The listing builds one solid part. Answer for the finished solid, in the listing's coordinates (mm). Face numbers are marked on the shaded views. A direction names the side the tool comes from. Round coordinates to 2 decimals unless told otherwise and drop trailing zeros. Order: outer loops, then holes, each group sorted by start corner. A loop starts at its lowest first (then second) coordinate and runs counter-clockwise, first axis right, second up. Notation, with made-up numbers: M 0.25,66.25 L 42.25,66.25 A28 ccw 42.25,92.25 Z; hole C 54.25,70.5 d7. An arc over 180 degrees is marked long. Put each result on its own line as item: value. Start each with the question number.
1. The part is cut by section D-D (z = 13). Give the vertices of the cut face in (x, y), then the cut area to 3 significant figures.
2. Which of the six approach directions +Z, -Z, +X, -X, +Y, -Y give full straight-line access (tool end or side, diameter ignored) to the marked faces 1, 2 and 3?
3. The part is cut by section B-B (x = 4). Give the vertices of the cut face in (y, z).
4. The mould has two halves that part along Y. Classify the marked faces 4, 5 and 6: +Y half, -Y half, draft (parallel to the pull), parting line (faces both ways), or undercut.
5. The part is cut by section A-A (z = 7). Give the vertices of the cut face in (x, y), then the cut area to 3 significant figures.
6. Consider line 1 (X direction, y = -12, z = 7); line 2 (Y direction, x = 2.25, z = 7); line 3 (X direction, y = 14.5, z = 12.75). Determine where each line is inside the solid, lowest interval first.
7. The part is cut by section C-C (y = 13). Give the vertices of the cut face in (x, z), then the cut area to 3 significant figures.
8. Each of these flat-tipped pins is pushed along its axis until it touches: pin 1 Ø4 at (x, z) = (23.01, 7) entering from -Y; pin 2 Ø6.5 at (y, z) = (14.35, 7) entering from +X; pin 3 Ø3 at (x, z) = (-5.5, 5) entering from +Y. Where does it stop, or does it pass through?
from build123d import *

# Parameters (mm, degrees)
SALIENTE_EXTRUIR1_DEPTH = 14
CROQUIS2_R              = 4.035649311
CORTAR_EXTRUIR1_DEPTH   = 14
CROQUIS5_R              = 2.497749653
CORTAR_EXTRUIR2_DEPTH   = 14
CROQUIS7_R              = 2.514867633
CORTAR_EXTRUIR3_DEPTH   = 14
CROQUIS8_W              = 1.02892534
CROQUIS8_H              = 10.439450899
CORTAR_EXTRUIR4_DEPTH   = 14
CROQUIS9_R              = 2.593975345
CORTAR_EXTRUIR5_DEPTH   = 30


with BuildPart() as part:
    # Croquis1 → Saliente-Extruir1 (new body)
    with BuildSketch(Plane.XY):
        Polygon((-2.000386176, 17.69916911), (15.999613824, 17.69916911), (15.999613824, -9.30083089), (26.999613824, -9.30083089), (26.999613824, -15.30083089), (15.999613824, -15.30083089), (-2.000386176, -15.30083089), (-13.000386176, -15.30083089), (-13.000386176, -9.30083089), (-2.000386176, -9.30083089), align=None)
    extrude(amount=SALIENTE_EXTRUIR1_DEPTH)

    # Croquis2 → Cortar-Extruir1 (cut)
    with BuildSketch(Plane.XY.offset(14)):
        with Locations((6.999613824, 4.803097651)):
            Circle(CROQUIS2_R)
    extrude(amount=-CORTAR_EXTRUIR1_DEPTH, mode=Mode.SUBTRACT)

    # Croquis5 → Cortar-Extruir2 (cut)
    with BuildSketch(Plane(origin=(0, -9.30083089, 0), x_dir=(1, 0, 0), z_dir=(0, 1, 0))):
        with Locations((-9.06576441, -7)):
            Circle(CROQUIS5_R)
    extrude(amount=-CORTAR_EXTRUIR2_DEPTH, mode=Mode.SUBTRACT)

    # Croquis7 → Cortar-Extruir3 (cut)
    with BuildSketch(Plane(origin=(0, -9.30083089, 0), x_dir=(1, 0, 0), z_dir=(0, 1, 0))):
        with Locations((23.014515722, -7)):
            Circle(CROQUIS7_R)
    extrude(amount=-CORTAR_EXTRUIR3_DEPTH, mode=Mode.SUBTRACT)

    # Croquis8 → Cortar-Extruir4 (cut)
    with BuildSketch(Plane.XY.offset(14)):
        with Locations((6.999613824, 13.435682)):
            Rectangle(CROQUIS8_W, CROQUIS8_H)
    extrude(amount=-CORTAR_EXTRUIR4_DEPTH, mode=Mode.SUBTRACT)

    # Croquis9 → Cortar-Extruir5 (cut, through all)
    with BuildSketch(Plane.ZY.offset(2.000386176)):
        with Locations((7, 14.351263228)):
            Circle(CROQUIS9_R)
    extrude(amount=-CORTAR_EXTRUIR5_DEPTH, mode=Mode.SUBTRACT)


solid = part.part
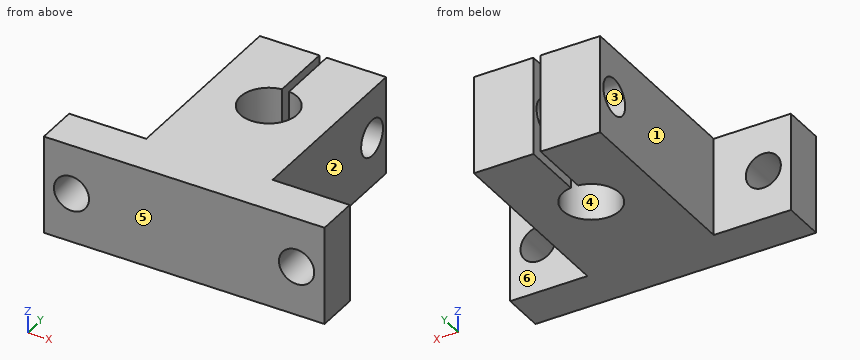
Resolved:
1. outline: M -13,-15.3 L 27,-15.3 L 27,-9.3 L 16,-9.3 L 16,17.7 L 7.51,17.7 L 7.51,8.81 A4.04 cw long 6.49,8.81 L 6.49,17.7 L -2,17.7 L -2,-9.3 L -13,-9.3 Z
1. area: 666 mm2
2. face 1: +Z, -Z, -X, +Y
2. face 2: +Z, -Z, +X, +Y
2. face 3: +X, -X
3. outline: M -15.3,0 L 2.1,0 L 2.1,14 L -15.3,14 Z; M 7.5,0 L 17.7,0 L 17.7,14 L 7.5,14 Z; hole C 14.35,7 d5.19
4. face 4: undercut
4. face 5: -Y half
4. face 6: +Y half
5. outline: M -13,-15.3 L -11.56,-15.3 L -11.56,-9.3 L -13,-9.3 Z; M -6.57,-15.3 L 20.5,-15.3 L 20.5,-9.3 L 16,-9.3 L 16,11.76 L 7.51,11.76 L 7.51,8.81 A4.04 cw long 6.49,8.81 L 6.49,11.76 L -2,11.76 L -2,-9.3 L -6.57,-9.3 Z; M -2,16.95 L 6.49,16.95 L 6.49,17.7 L -2,17.7 Z; M 7.51,16.95 L 16,16.95 L 16,17.7 L 7.51,17.7 Z; M 25.53,-15.3 L 27,-15.3 L 27,-9.3 L 25.53,-9.3 Z
5. area: 518 mm2
6. line 1: -13 to -11.56, -6.57 to 20.5, 25.53 to 27
6. line 2: -15.3 to 11.76, 16.95 to 17.7
6. line 3: -2 to 6.49, 7.51 to 16
7. outline: M -2,0 L 6.49,0 L 6.49,4.79 L -2,4.79 Z; M -2,9.21 L 6.49,9.21 L 6.49,14 L -2,14 Z; M 7.51,0 L 16,0 L 16,4.79 L 7.51,4.79 Z; M 7.51,9.21 L 16,9.21 L 16,14 L 7.51,14 Z
7. area: 162 mm2
8. pin 1: through
8. pin 2: x = 16
8. pin 3: y = -9.3
